CAD build for the part. Positions are in the model's coordinates, mm. A direction names the side the tool comes from. Give positions to 0.01 mm unless a question says otherwise; leave off trailing zeros. Order: outer loops, then holes, each group sorted by start corner. A loop starts at its lowest first (then second) coordinate and runs counter-clockwise, first axis right, second up.
Item 1: Band-saw the part on D-D on z = -18. Give the cut face in (x, y).
Item 2: Which spindle directions (+Z, -Z, +X, -X, +Y, -Y) get a long thin tool onto all of the face, cutting with end or side? Do faces 5 (the flat face through (0.1, -12.2, 0)), 6 (the cylindrical face through (22.68, -0.07, -1.57)), 7 (the flat face through (17, -3.175, -2)), 8 (the flat face through (-17, 3.175, -2)), 9 (the flat face through (17, 3.175, -2)). Say none if no direction does.
Item 3: Two-plate mould, pull along X, no slides. Class faces 1 (the cylindrical face through (-9.45, -7.24, -11.11)), 2 (the cylindrical face through (17.875, 0.072, -1.565)), 3 (the flat face through (-17, -3.175, -2)), 4 (the cylindrical face through (-22.68, -0.07, -1.57)): released by +X, released by -X, zero draft, split by the parting line, or undercut.
Item 4: Flat gauge pins, fed straight in: P1, Ø2.5, axis at x = 17.5, z = -1.5, coming from the +Y side (3 decimals); P2, Ø4, axis at x = -19.51, y = 0, coming from the -Z side (3 decimals); P3, Ø1.6, axis at x = -17, z = -2, coming from the -Y side (3 decimals). Where does each tip first touch, or does it go through?
Item 5: Band-saw the part on C-C on y = -6.5. Give the cut face in (x, z).
Item 6: Band-saw the part on A-A on x = 0. Give the cut face in (y, z), plus the area to 3 significant figures.
Item 7: Wall check: L1, parallel to Z at x = -15.5, y = -2 (3 decimals); L2, parallel to X at y = -8, z = -4.5; L3, parallel to Y at x = 9.5, z = -2.75. Give the ranges that are in metal, low to high.
Item 8: Band-saw the part on B-B on y = 0. Give the cut face in (x, z) (1 decimal), plus the area to 3 significant figures.
```python
from build123d import *

# Parameters (mm, degrees)
F0_R     = 15.08125
F0_R_2   = 11.90625
F1_DEPTH = 22.5425
F2_R     = 1.63195
F3_DEPTH = 3.175


# Not quite as in the source:
# - a pattern or mirror of a feature is missing from the dataset's text; its kind, count and spacing are read off the source's solid


with BuildPart() as f1:
    # F0 (on Top) → F1 (new body)
    with BuildSketch(Plane.XY):
        Circle(F0_R)
        Circle(F0_R_2, mode=Mode.SUBTRACT)
    extrude(amount=-F1_DEPTH)

    # F2 (on Top) → F3 (join)
    with BuildSketch(Plane.XY):
        with BuildLine():
            Line((19.5057518992, 3.175), (14.7432518992, 3.175))
            Line((14.7432518992, 3.175), (14.7432518992, -3.175))
            Line((14.7432518992, -3.175), (19.5057518992, -3.175))
            ThreePointArc((19.5057518992, -3.175), (22.6807518992, 0), (19.5057518992, 3.175))
        make_face()
        with Locations((19.5057518992, 0)):
            Circle(F2_R, mode=Mode.SUBTRACT)
    f3 = extrude(amount=-F3_DEPTH)

    # F3_copies: F3 across plane
    add(f3.mirror(Plane(origin=(0, 0, 0), x_dir=(0, 0, -1), z_dir=(-1, 0, 0))))


solid = f1.part
```
The answers:
1. outline: circle Ø30.16 at (0, 0); hole circle Ø23.81 at (0, 0)
2. face 5: +Z, +X, -X, +Y, -Y
2. face 6: +Z, -Z, +X
2. face 7: +Z, -Z, +X, -Y
2. face 8: +Z, -Z, -X, +Y
2. face 9: +Z, -Z, +X, +Y
3. face 1: undercut
3. face 2: undercut
3. face 3: zero draft
3. face 4: released by -X
4. P1: stops at y = 3.175
4. P2: stops at z = -3.175
4. P3: stops at y = -3.175
5. outline: (-13.61, -22.54) - (-9.98, -22.54) - (-9.98, 0) - (-13.61, 0) - close; (9.98, -22.54) - (13.61, -22.54) - (13.61, 0) - (9.98, 0) - close
6. outline: (-15.08, -22.54) - (-11.91, -22.54) - (-11.91, 0) - (-15.08, 0) - close; (11.91, -22.54) - (15.08, -22.54) - (15.08, 0) - (11.91, 0) - close
6. area: 143 mm2
7. L1: z = -3.175 to 0
7. L2: x = -12.78 to -8.82, 8.82 to 12.78
7. L3: y = -11.71 to -7.18, 7.18 to 11.71
8. outline: (-22.7, -3.2) - (-21.1, -3.2) - (-21.1, 0) - (-22.7, 0) - close; (-17.9, -3.2) - (-15.1, -3.2) - (-15.1, -22.5) - (-11.9, -22.5) - (-11.9, 0) - (-17.9, 0) - close; (11.9, -22.5) - (15.1, -22.5) - (15.1, -3.2) - (17.9, -3.2) - (17.9, 0) - (11.9, 0) - close; (21.1, -3.2) - (22.7, -3.2) - (22.7, 0) - (21.1, 0) - close
8. area: 171 mm2
